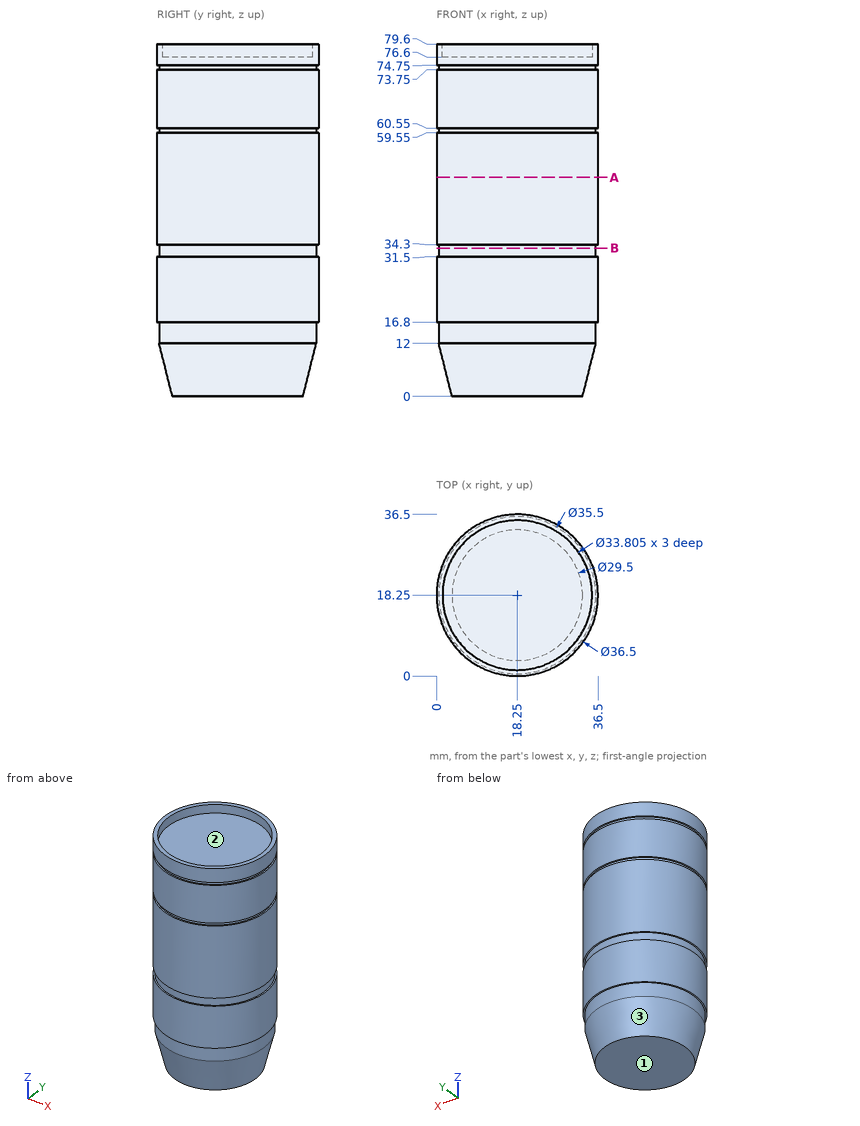
Geometry: see drawing. Coordinates: mm, zero at the bounding-box minimum. Coordinates: 2 decimals unless noted, no trailing zeros. Loops run counter-clockwise (first coordinate to the right, second up) from the corner with the lowest first, then second, coordinate; pieces in that order, holes last.
Q1. Cut plane B-B (z = 33.5). Output: boundary loops of the cut face in (x, y).
Q2. Draft query along Y for the marked faces 1, 2 and 3. Return one class per face: +Y half, -Y half, draft (parallel to the pull), parting line (faces both ways), or undercut.
Q3. Cut plane A-A (z = 49.5). Output: boundary loops of the cut face in (x, y).
Q4. Contact query for flat-ended pins moving along their axis: pin 1 (18 mm diameter, centred on x = 23, y = 15, fed in from +Z); pin 2 (12 mm diameter, centred on y = 31.5, z = 66, fed in from -X); pin 3 (2 mm diameter, centred on x = 5, z = 67, fed in from +Y). Output: stop coordinate, or through.
Q5. Material intervals for line 1 (X direction, y = 18, z = 77); line 2 (Y direction, x = 18, z = 75), sorted ascending.
Working result:
1. outline: circle Ø35.5 at (18.25, 18.25)
2. face 1: draft
2. face 2: undercut
2. face 3: parting line
3. outline: circle Ø36.5 at (18.25, 18.25)
4. pin 1: stops at z = 76.6
4. pin 2: stops at x = 1.5
4. pin 3: stops at y = 31.78
5. line 1: x = 0 to 1.35, 35.15 to 36.5
5. line 2: y = 0 to 36.5
